Build history of the part. All positions in model axes, mm. Face numbers are marked on the shaded views. A direction names the side the tool comes from. Coordinates: 2 decimals unless noted, no trailing zeros. Write each loop counter-clockwise with the first axis right and the second up, starting at its lowest first coordinate (ties: lowest second). Pieces come first, ordered by that corner, then holes. Notation, with made-up numbers: M 47.5,11 L 65.5,11 A15 ccw 65.5,34 Z; hole C -11,-25.75 d3. An arc over 180 degrees is marked long. Use CSV: the item, a comma, the result in double quotes. Start each with the question number.
Autodesk Inventor part; units mm, degrees
ref_plane "Work Plane1" through (0, 0.2, -0.3) normal (0, 0, 1) x (1, 0, 0)
ref_plane "YZ Plane" through (0, 0, 0) normal (1, 0, 0) x (0, 1, 0)
ref_plane "XZ Plane" through (0, 0, 0) normal (0, 1, 0) x (-1, 0, 0)
sketch "Sketch1" plane through (0, 0, 0) normal (1, 0, 0) x (0, 1, 0)
  line L0 (1.1156, 6.8012) -> (0.4531, 6.6963)
  line L1 (0.4531, 6.1037) -> (1.1156, 5.9988)
  line L2 (1.2, 5.9) -> (1.2, 0.1)
  line L3 (1.1, 0) -> (0.3, 0)
  line L4 (0, -0.3) -> (0, -2.6)
  line L5 (-0.3, -2.9) -> (-5.95, -2.9)
  line L6 (-5.95, -2.9) -> (-5.95, -3.1)
  line L7 (-5.95, -3.1) -> (-0.3, -3.1)
  line L8 (0.2, -2.6) -> (0.2, -0.3)
  line L9 (0.3, -0.2) -> (1.1, -0.2)
  line L10 (1.4, 0.1) -> (1.4, 5.9)
  line L11 (1.1469, 6.1963) -> (0.4844, 6.3012)
  line L12 (0.4844, 6.4988) -> (1.1469, 6.6037)
  line L13 (1.4, 6.9) -> (1.4, 7.65)
  line L14 (1.4, 7.65) -> (1.2, 7.65)
  line L15 (1.2, 7.65) -> (1.2, 6.9)
  line L16 (0, -5.3743) -> (0, 9.8207)
  line L17 (-7.4324, 0) -> (2.9446, 0)
  arc A0 (0.3, -0.2) -> (0.2, -0.3) centre (0.3, -0.3) ccw
  arc A1 (-0.3, -2.9) -> (0, -2.6) centre (-0.3, -2.6) ccw
  arc A2 (1.1, 0) -> (1.2, 0.1) centre (1.1, 0.1) ccw
  arc A3 (1.2, 5.9) -> (1.1156, 5.9988) centre (1.1, 5.9) ccw
  arc A4 (0.4844, 6.4988) -> (0.4844, 6.3012) centre (0.5, 6.4) ccw
  arc A5 (1.1156, 6.8012) -> (1.2, 6.9) centre (1.1, 6.9) ccw
  arc A6 (0.4531, 6.6963) -> (0.4531, 6.1037) centre (0.5, 6.4) ccw
  arc A7 (1.4, 5.9) -> (1.1469, 6.1963) centre (1.1, 5.9) ccw
  arc A8 (1.1469, 6.6037) -> (1.4, 6.9) centre (1.1, 6.9) ccw
  arc A9 (1.1, -0.2) -> (1.4, 0.1) centre (1.1, 0.1) ccw
  arc A10 (0.3, 0) -> (0, -0.3) centre (0.3, -0.3) ccw
  arc A11 (-0.3, -3.1) -> (0.2, -2.6) centre (-0.3, -2.6) ccw
  point P0 (1.2, 6.8146)
  point P1 (0, -2.9)
  point P2 (1.4, 6.1562)
  point P3 (-0.1393, 6.4)
  point P4 (1.4, 6.6438)
  dimension "d0" = 0.2
  dimension "d1" = 0.2
  dimension "d3" = 0.2
  dimension "d8" = 0.2
  dimension "d9" = 0.2
  dimension "d10" = 0.2
  dimension "d12" = 5.95
  dimension "d16" = 1.2
  dimension "d20" = 0.2438
  dimension "d21" = 0.2438
  dimension "d23" = 0.1
  dimension "d25" = 1
  dimension "d26" = 9.8
  dimension "d27" = 0.75
  dimension "d28" = 2.6
  dimension "d31" = 9.3
  dimension "d70" = 0.3
extrude "Extrusion1" add sketch "Sketch1" along normal blind 1.7 contours A5 L15 L14 L13 A8 L12 A4 L11 A7 L10 A9 L17 A2 L2 A3 L1 A6 L0 | L17 A9 L9 A0 L8 A11 L16 L4 A10 L3 | L16 A11 L7 L6 L5 A1
ref_plane "Work Plane1" through (0, 0.2, -0.3) normal (0, 0, 1) x (1, 0, 0)
sketch "Sketch2" plane through (0, 0.3, -0.3) normal (0, 0, -1) x (-1, 0, 0)
  line L0 (0, 1.1) -> (-1.7, 1.1)
  line L1 (0, -0.3) -> (-1.7, -0.3)
  line L2 (-1.35, 1.1) -> (-0.35, 1.1)
  line L3 (-0.35, 1.1) -> (-0.35, -0.3)
  line L4 (-0.35, -0.3) -> (-1.35, -0.3)
  line L5 (-1.35, -0.3) -> (-1.35, 1.1)
  line L6 (-1.7, 0) -> (-1.7, 0.8)
  line L7 (0, 0) -> (0, 0.8)
  line L8 (-1.7, 0) -> (-1.7, -0.3)
  line L9 (-1.35, 1.1) -> (-1.7, 1.1)
  line L10 (-1.7, 1.1) -> (-1.7, -0.3)
  line L11 (-1.7, -0.3) -> (-1.35, -0.3)
  line L12 (-1.35, -0.3) -> (-1.35, 1.1)
  line L13 (0, 0) -> (0, -0.3)
  line L14 (-0.35, 1.1) -> (0, 1.1)
  line L15 (0, 1.1) -> (0, -0.3)
  line L16 (0, -0.3) -> (-0.35, -0.3)
  line L17 (-0.35, -0.3) -> (-0.35, 1.1)
  dimension "d32" = 1
  dimension "d33" = 0.35
  dimension "d34" = 0.35
extrude "Extrusion2" cut sketch "Sketch2" against normal up to surface (7.95 mm away) contours L15 L7 L13 L1 L3 L0 | L5 L1 L8 L6 L10 L0
sketch "Sketch3" plane through (0, 0.2, -2.6) normal (0, 1, 0) x (1, 0, 0)
  line L0 (0.35, -2.3) -> (1.35, -2.3)
  line L1 (1.35, -2.3) -> (1.7, -1.6938)
  line L2 (1.7, 0) -> (1.7, -2.3)
  line L3 (1.35, -2.3) -> (2.05, -2.3) construction
  line L4 (1.7, -1.6938) -> (1.7, -2.3)
  line L5 (1.35, -2.3) -> (1.7, -2.3)
  line L6 (1.7, -2.3) -> (1.35, -2.3)
  line L7 (1.35, -2.3) -> (0.35, -2.3)
  line L8 (0, -2.3) -> (0, 0)
  line L9 (0.35, -2.3) -> (0, -2.3)
  line L10 (0, -2.3) -> (0, -1.6938)
  line L11 (0, -1.6938) -> (0.35, -2.3)
  line L12 (0.35, -0.3) -> (0.35, 0.3)
  line L13 (1.35, -0.3) -> (1.7, -0.3)
  line L14 (1.7, -0.3) -> (1.7, 0.5)
  line L15 (1.7, 0.5) -> (1.35, 0.5)
  line L16 (1.35, 0.5) -> (1.35, -0.3)
  line L17 (0.35, -0.3) -> (0, -0.3)
  line L18 (0, -0.3) -> (0, 0.5)
  line L19 (0, 0.5) -> (0.35, 0.5)
  line L20 (0.35, 0.5) -> (0.35, -0.3)
  line L21 (0, 0) -> (1.7, 0)
  point P0 (0, -2.6)
  point P1 (0, -1.6938)
  point P2 (0.35, 0.3)
  point P3 (0.35, 0.3)
  dimension "d38" = 60
  dimension "d39" = 60
  dimension "d59" = 2
  dimension "d60" = 2
  dimension "d62" = 1
  dimension "d63" = 0.35
  dimension "d64" = 0.35
extrude "Extrusion3" cut sketch "Sketch3" against normal up to surface (6.15 mm away) contours L9 L8 L11 | L1 L2 L5 | L8 L21 L12 L17 | L13 L16 L21 L2 | L18 L19 L20 L12 L21 | L21 L16 L15 L14
sketch "Sketch5" plane through (1.35, -0.3, -3.1) normal (0, 0, -1) x (-1, 0, 0)
  line L0 (0, -1.15) -> (0.25, -1.4)
  line L1 (0.25, -1.4) -> (0.25, -5.317)
  line L2 (0.25, -5.317) -> (0.4134, -5.6)
  line L3 (0.5866, -5.6) -> (0.75, -5.317)
  line L4 (0.75, -5.317) -> (0.75, -1.4)
  line L5 (0.75, -1.4) -> (1, -1.15)
  line L6 (0.25, -5.317) -> (0.75, -5.317) construction
  line L7 (0, -1.15) -> (1, -1.15) construction
  arc A0 (0.4134, -5.6) -> (0.5866, -5.6) centre (0.5, -5.55) ccw
  line L8 (0, 0.3) -> (-0.35, 0.3)
  line L9 (1.35, 0.3) -> (1, 0.3)
  line L10 (0, 0) -> (0, -5.65)
  line L11 (1, -5.65) -> (1, 0)
  line L12 (1, -5.65) -> (0, -5.65)
  point P0 (0.5, -5.65)
  point P1 (1.35, -5.85)
  point P2 (-0.35, -5.85)
  point P3 (0, 0.6)
  point P4 (1, 0.6)
  point P5 (0.5, -5.35)
  dimension "d45" = 60
  dimension "d46" = 0.5
  dimension "d48" = 135
  dimension "d49" = 135
  dimension "d53" = 0.1
  dimension "d65" = 1.7
  dimension "d66" = 1.7
  dimension "d67" = 0.25
  dimension "d68" = 0.5
  dimension "d69" = 0.25
extrude "Extrusion4" cut sketch "Sketch5" against normal up to surface (0.2 mm away)
equation "\"d33\" = d34"
equation "\"d63\" = d64"
equation "\"BendRadius\" = Thickness"
equation "\"BendReliefWidth\" = Thickness"
equation "\"BendReliefDepth\" = 0.5 * Thickness"
equation "\"CornerReliefSize\" = 4 * Thickness"
equation "\"MinimumRemnant\" = 2 * Thickness"
equation "\"TransitionRadius\" = BendRadius"
equation "\"JacobiRadiusSize\" = BendRadius"
equation "\"GapSize\" = Thickness"
properties part number "USB 3.0 A Recepticle Lower Pin" material "Nickel-Copper Alloy 400"
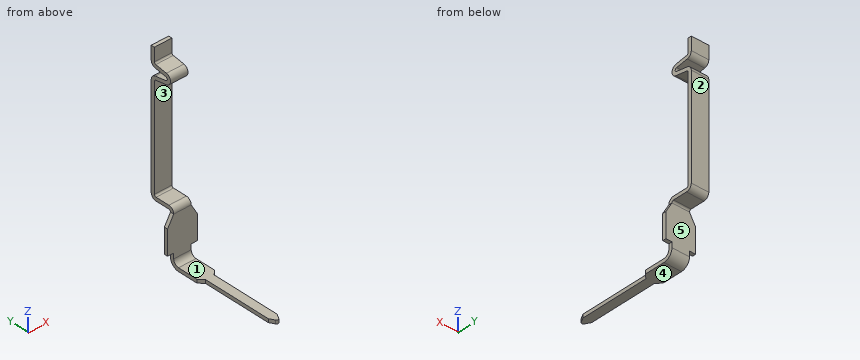
1. Flat gauge pins, fed straight in: pin 1 (0.5 mm diameter, centred on x = 0.5, z = -2, fed in from +Y); pin 2 (0.8 mm diameter, centred on x = 0.5, z = 7.5, fed in from -Y); pin 3 (1 mm diameter, centred on x = 1, y = -4.5, fed in from +Z). Where does each tip first touch, or does it go through?
2. Drill centre lines: line 1 along Z through (x, y) = (1.1, -1.25); line 2 along X through (y, z) = (1.25, 3); line 3 along Z through (x, y) = (1.3, 0.5). Where is each one in solid material? Low to high. Write a range as from..to.
3. Pull direction Z, two halves, no side cores. Call the marked faces 3, 4 and 5: pulls with the +Z half, pulls with the -Z half, needs draft (parallel to the pull), parting line crosses it, or undercut.
4. Slice it at A-A (z = -1.75). List the corners of the cut face in (x, y).
5. 3-axis set-ups, long thin cutter, end or side, ignore diameter. For the marked faces 1 and 2: which of +Z, -Z, +X, -X, +Y, -Y reach the whole face in a straight line?
6. Slice it at B-B (y = -2). List the corners of the cut face in (x, z), and give its area (3 significant figures).
Established:
1,pin 1,"stops at y = 0.2"
1,pin 2,"stops at y = 1.2"
1,pin 3,"stops at z = -2.9"
2,line 1,"z = -3.1..-2.9"
2,line 2,"x = 0.35..1.35"
2,line 3,"z = -0.2..0, 6.1..6.3, 6.5..6.7"
3,face 3,"undercut"
3,face 4,"pulls with the -Z half"
3,face 5,"needs draft"
4,outline,"M 0,0 L 1.7,0 L 1.7,0.2 L 0,0.2 Z"
5,face 1,"+Z, +X, -X, -Y"
5,face 2,"+Z, -Z, +X, -X, +Y"
6,outline,"M 0.6,-3.1 L 1.1,-3.1 L 1.1,-2.9 L 0.6,-2.9 Z"
6,area,"0.100 mm2"
